Verification items for the finished model (mm, model axes). A direction names the side the tool comes from. Coordinates: 2 decimals unless noted, no trailing zeros. Loops run counter-clockwise (first coordinate to the right, second up) from the corner with the lowest first, then second, coordinate; pieces in that order, holes last.
Q1. Sectioned sample at B-B (y = 12). Enter the section's corners in (x, z), then the cut area to 3 significant figures.
Q2. Sectioned sample at D-D (x = -5). Enter the section's corners in (y, z).
Q3. Access from +Z, -Z, +X, -X, +Y, -Y to the whole of each face (thin tool, end or side, straight path). Record for faces 4 (the face through (-9, -10, 11)), 5 (the face through (-12, -10, 4)), 6 (the face through (-20, 5, 8)), 7 (the face through (12, 67, 2)), 8 (the face through (-0.325, -11.464, 22.425)).
Q4. Sectioned sample at A-A (z = 14.75). Enter the section's corners in (x, y), then the cut area to 3 significant figures.
Q5. Material ranges on probe 1 along X at (y, z) = (-10, 6.75); probe 2 along Y at (x, z) = (0, 22.2); probe 3 along Y at (x, z) = (22.5, 5), recorded low to high.
Q6. Mould release check, pull along Z, two halves, no side actions. Record for faces 1 (the face through (23.196, 10.07, 10.169)), 2 (the face through (3.564, 36.856, 0.927)), 3 (the face through (0, -7, 23.13)): +Z half, -Z half, draft (parallel to the pull), parting line (faces both ways), or undercut.
Q7. Go/stop test with flat-tipped pins: P1, Ø2, axis at x = 16, z = 10, coming from the +Y side; P2, Ø1.5, axis at y = 6.5, z = 11.5, coming from the +X side; P3, Ø3, axis at x = -18, z = 5, coming from the +Y side; P4, Ø10, axis at x = 9.5, z = 21.5, coming from the +Y side. Record where each tip stops, or that it passes through.
Q8. Sectioned sample at C-C (z = 9.25). Enter the section's corners in (x, y).
```python
from build123d import *

# Parameters (mm, degrees)
SALIENTE_EXTRUIR1_DEPTH = 1.88
SALIENTE_EXTRUIR2_DEPTH = 4.03
REDONDEO1_R             = 2
CROQUIS3_W              = 13
CROQUIS3_H              = 10
SALIENTE_EXTRUIR3_DEPTH = 10
REDONDEO2_R             = 6
CROQUIS4_W              = 18
CROQUIS4_H              = 10
SALIENTE_EXTRUIR4_DEPTH = 24
CHAFL_N1_SIZE           = 5
CORTAR_EXTRUIR1_DEPTH   = 24
CROQUIS6_R              = 1.5
CORTAR_EXTRUIR2_DEPTH   = 14
CROQUIS7_W              = 3
CROQUIS7_H              = 1.5
CORTAR_EXTRUIR3_DEPTH   = 14
CROQUIS8_R              = 2.5
CORTAR_EXTRUIR4_DEPTH   = 65.060708707


with BuildPart() as part:
    # Croquis1 → Saliente-Extruir1 (new body)
    with BuildSketch(Plane.XY):
        with BuildLine():
            Line((-11, 15), (-11, 68))
            Line((-11, 68), (12, 68))
            Line((12, 68), (12, 65.5))
            Line((12, 65.5), (-1.3, 65.5))
            ThreePointArc((-1.3, 65.5), (-3.067766953, 64.767766953), (-3.8, 63))
            Line((-3.8, 63), (-3.8, 58.913644565))
            ThreePointArc((-3.8, 58.913644565), (-3.7664666, 58.505548363), (-3.666765992, 58.108400044))
            Line((-3.666765992, 58.108400044), (11, 15))
            Line((11, 15), (25, 15))
            Line((25, 15), (25, -15))
            Line((25, -15), (-25, -15))
            Line((-25, -15), (-25, 15))
            Line((-25, 15), (-11, 15))
        make_face()
        with BuildLine():
            Line((-6, 10), (-6, 49.44298114))
            Line((-6, 49.44298114), (7.419680939, 10))
            ThreePointArc((7.419680939, 10), (0.70984047, 3.29015953), (-6, 10))
        make_face(mode=Mode.SUBTRACT)
    extrude(amount=SALIENTE_EXTRUIR1_DEPTH)

    # Croquis2 → Saliente-Extruir2 (add)
    with BuildSketch(Plane.XY.offset(1.88)):
        Polygon((-1.3, 65.5), (-11, 65.5), (-11, 68), (12, 68), (12, 65.5), align=None)
    extrude(amount=SALIENTE_EXTRUIR2_DEPTH)

    # Redondeo1
    redondeo1_edges = [part.edges().sort_by_distance(p)[0] for p in [
        (-11, 66.75, 5.91),
        (12, 66.75, 5.91),
    ]]
    fillet(redondeo1_edges, radius=REDONDEO1_R)

    # Croquis3 → Saliente-Extruir3 (add)
    with BuildSketch(Plane.XY.offset(1.88)):
        with Locations((-18.5, 10)):
            Rectangle(CROQUIS3_W, CROQUIS3_H)
        with Locations((-18.5, -10)):
            Rectangle(CROQUIS3_W, CROQUIS3_H)
        with Locations((18.5, -10)):
            Rectangle(CROQUIS3_W, CROQUIS3_H)
        with Locations((18.5, 10)):
            Rectangle(CROQUIS3_W, CROQUIS3_H)
    extrude(amount=SALIENTE_EXTRUIR3_DEPTH)

    # Redondeo2
    redondeo2_edges = [part.edges().sort_by_distance(p)[0] for p in [
        (25, -10, 11.88),
        (12, -10, 11.88),
        (25, 10, 11.88),
        (12, 10, 11.88),
        (-25, 10, 11.88),
        (-12, 10, 11.88),
        (-25, -10, 11.88),
        (-12, -10, 11.88),
    ]]
    fillet(redondeo2_edges, radius=REDONDEO2_R)

    # Croquis4 → Saliente-Extruir4 (add)
    with BuildSketch(Plane.XY.offset(1.88)):
        with Locations((0, -10)):
            Rectangle(CROQUIS4_W, CROQUIS4_H)
    extrude(amount=SALIENTE_EXTRUIR4_DEPTH)

    # Chaflán1
    chafl_n1_edges = [part.edges().sort_by_distance(p)[0] for p in [
        (9, -10, 25.88),
        (-9, -10, 25.88),
    ]]
    chamfer(chafl_n1_edges, length=CHAFL_N1_SIZE)

    # Croquis5 → Cortar-Extruir1 (cut)
    with BuildSketch(Plane(origin=(0, -5, 0), x_dir=(1, 0, 0), z_dir=(0, 1, 0))):
        with BuildLine():
            Line((0, -7.895), (-3.968626967, -11.395))
            ThreePointArc((-3.968626967, -11.395), (0, -21.895), (3.968626967, -11.395))
            Line((3.968626967, -11.395), (0, -7.895))
        make_face()
    extrude(amount=-CORTAR_EXTRUIR1_DEPTH, mode=Mode.SUBTRACT)

    # Croquis6 → Cortar-Extruir2 (cut)
    with BuildSketch(Plane.XY.offset(25.88)):
        with Locations((0, -10)):
            Circle(CROQUIS6_R)
    extrude(amount=-CORTAR_EXTRUIR2_DEPTH, mode=Mode.SUBTRACT)

    # Croquis7 → Cortar-Extruir3 (cut)
    with BuildSketch(Plane(origin=(0, -5, 0), x_dir=(1, 0, 0), z_dir=(0, 1, 0))):
        with Locations((0, -23.88)):
            Rectangle(CROQUIS7_W, CROQUIS7_H)
    extrude(amount=-CORTAR_EXTRUIR3_DEPTH, mode=Mode.SUBTRACT)

    # Croquis8 → Cortar-Extruir4 (cut, through all)
    with BuildSketch(Plane(origin=(0, 15, 0), x_dir=(1, 0, 0), z_dir=(0, 1, 0))):
        with Locations(Location((-18.5, -5.45, 0), (0, 0, 180))):
            Circle(CROQUIS8_R)
        with Locations(Location((18.5, -5.45, 0), (0, 0, 180))):
            Circle(CROQUIS8_R)
    extrude(amount=-CORTAR_EXTRUIR4_DEPTH, mode=Mode.SUBTRACT)


solid = part.part
```
Geometry check:
1. outline: (-25, 0) - (-6, 0) - (-6, 1.88) - (-12, 1.88) - (-12, 5.88) arc R6 ccw to (-18, 11.88) - (-19, 11.88) arc R6 ccw to (-25, 5.88) - close; (6.74, 0) - (25, 0) - (25, 5.88) arc R6 ccw to (19, 11.88) - (18, 11.88) arc R6 ccw to (12, 5.88) - (12, 1.88) - (6.74, 1.88) - close; hole circle Ø5 at (-18.5, 5.45); hole circle Ø5 at (18.5, 5.45)
1. area: 260 mm2
2. outline: (-15, 0) - (6.48, 0) - (6.48, 1.88) - (-5, 1.88) - (-5, 12.58) - (-15, 12.58) - close; (-15, 19.21) - (-5, 19.21) - (-5, 24.88) - (-15, 24.88) - close; (46.5, 0) - (68, 0) - (68, 5.91) - (65.5, 5.91) - (65.5, 1.88) - (46.5, 1.88) - close
3. face 4: +Z, -Y
3. face 5: +Z, +Y, -Y
3. face 6: +Z, +X, -X
3. face 7: +Z, -Z, +X, +Y
3. face 8: +Z
4. outline: (-9, -15) - (-5.89, -15) - (-5.89, -5) - (-9, -5) - close; (5.89, -15) - (9, -15) - (9, -5) - (5.89, -5) - close
4. area: 62.2 mm2
5. probe 1: x = -24.94 to -20.64, -16.36 to -12.06, -9 to 9, 12.06 to 16.36, 20.64 to 24.94
5. probe 2: y = -15 to -11.5, -8.5 to -5
5. probe 3: y = -15 to -5, 5 to 15
6. face 1: +Z half
6. face 2: draft
6. face 3: undercut
7. P1: stops at y = 15
7. P2: stops at x = 22.5
7. P3: passes through
7. P4: stops at y = -5
8. outline: (-23.96, -15) - (-13.04, -15) - (-13.04, -5) - (-23.96, -5) - close; (-23.96, 5) - (-13.04, 5) - (-13.04, 15) - (-23.96, 15) - close; (-9, -15) - (-1.54, -15) - (-1.54, -5) - (-9, -5) - close; (1.54, -15) - (9, -15) - (9, -5) - (1.54, -5) - close; (13.04, -15) - (23.96, -15) - (23.96, -5) - (13.04, -5) - close; (13.04, 5) - (23.96, 5) - (23.96, 15) - (13.04, 15) - close
